The listing builds one solid part. Answer for the finished solid, in the listing's coordinates (mm). Face numbers are marked on the shaded views. A direction names the side the tool comes from. Round coordinates to 2 decimals unless told otherwise and drop trailing zeros. Write each loop counter-clockwise with the first axis right and the second up, starting at its lowest first coordinate (ties: lowest second). Pieces come first, ordered by that corner, then holes. Notation, with made-up numbers: (60.5, -33) - (116.5, -33) arc R32 ccw to (116.5, 5) - close; hole circle Ø1 at (-26.5, -2.5). An arc over 180 degrees is marked (long way). Return JSON: item names as keys, results as strings. Group by question number.
(1) Find the intervals of material crossed by line 1 along X through (y, z) = (0, 2); line 2 along Y through (x, z) = (0, 29.5) (3 decimals), in increasing order. Write a range as [from, to].
(2) Determine the mould class of the marked faces 1, 2 and 3 for opening direction Y: +Y half, -Y half, draft (parallel to the pull), parting line (faces both ways), or undercut.
(3) Section A-A, the plane x = 0 is taken. Write down the section's boundary in (y, z) (3 decimals), then the cut area to 3 significant figures.
(4) Each of these flat-tipped pins is pushed along its axis until it touches: pin 1 (10 mm diameter, centred on x = -16.5, z = 41, fed in from -Y); pin 2 (3 mm diameter, centred on x = -11.5, y = 0.5, fed in from -Z) (3 decimals); pin 3 (3 mm diameter, centred on y = 15.5, z = 7.5, fed in from -X). Where does it stop, or does it pass through?
(5) Section B-B, the plane z = 27 is taken. Write down the section's boundary in (x, y) (3 decimals), then the cut area to 3 significant figures.
(6) Section D-D, the plane z = 15 is taken. Write down the section's boundary in (x, y) (3 decimals).
(7) Which of the six approach directions +Z, -Z, +X, -X, +Y, -Y give full straight-line access (tool end or side, diameter ignored) to the marked faces 4 and 5?
```python
from build123d import *

# Parameters (mm, degrees)
F0_R        = 22.225
F1_DEPTH    = 63.5
F2_R        = 18.4381673654
F3_DEPTH    = 44.45
F4_R        = 22.225
F4_R_2      = 20.7260281568
F5_DEPTH    = 12.7
F6_R        = 14.6680324841
F1_FACE_R   = 22.225
F1_FACE_R_2 = 18.4381673654
F7_DEPTH    = 3.175


with BuildPart() as f1:
    # F0 (on Top) → F1 (new body)
    with BuildSketch(Plane.XY):
        Circle(F0_R)
    extrude(amount=F1_DEPTH)

    # F2 (on face) → F3 (cut)
    with BuildSketch(Plane.XY.offset(63.5)):
        Circle(F2_R)
    extrude(amount=-F3_DEPTH, mode=Mode.SUBTRACT)

    # F4 (on face) → F5 (cut)
    with BuildSketch(Plane(origin=(0, 0, 0), x_dir=(1, 0, 0), z_dir=(0, 0, -1))):
        Circle(F4_R)
        Circle(F4_R_2, mode=Mode.SUBTRACT)
    extrude(amount=-F5_DEPTH, mode=Mode.SUBTRACT)

    # F6 (on face) + F1_face (on face) → F7 (cut)
    with BuildSketch(Plane(origin=(0, 0, 0), x_dir=(1, 0, 0), z_dir=(0, 0, -1))):
        Circle(F6_R)
    with BuildSketch(Plane.XY.offset(63.5)):
        Circle(F1_FACE_R)
        Circle(F1_FACE_R_2, mode=Mode.SUBTRACT)
    extrude(amount=-F7_DEPTH, dir=(0, 0, -1), mode=Mode.SUBTRACT)


solid = f1.part
```
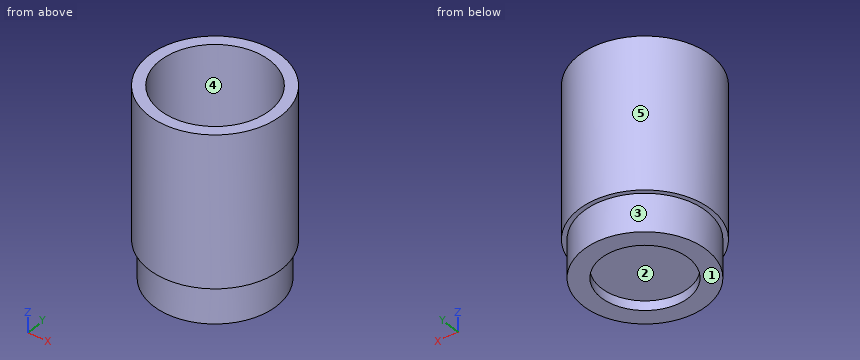
Working result:
{
 "1": {"line 1": "x = [-20.73, -14.67], [14.67, 20.73]", "line 2": "y = [-22.225, -18.438], [18.438, 22.225]"},
 "2": {"face 1": "draft", "face 2": "undercut", "face 3": "parting line"},
 "3": {"outline": "(-22.225, 12.7) - (-20.726, 12.7) - (-20.726, 0) - (-14.668, 0) - (-14.668, 3.175) - (14.668, 3.175) - (14.668, 0) - (20.726, 0) - (20.726, 12.7) - (22.225, 12.7) - (22.225, 63.5) - (18.438, 63.5) - (18.438, 19.05) - (-18.438, 19.05) - (-18.438, 63.5) - (-22.225, 63.5) - close", "area": "1,050 mm^2"},
 "4": {"pin 1": "stops at y = -19.02", "pin 2": "stops at z = 3.175", "pin 3": "stops at x = -15.28"},
 "5": {"outline": "circle Ø44.45 at (0, 0); hole circle Ø36.876 at (0, 0)", "area": "484 mm^2"},
 "6": {"outline": "circle Ø44.45 at (0, 0)"},
 "7": {"face 4": "+Z", "face 5": "+Z, -Z"}
}
